Design review of the part built by this model. Coordinates are the model's own, in mm. A direction names the side the tool comes from. Give positions to 0.01 mm unless a question says otherwise; leave off trailing zeros. Write each loop counter-clockwise with the first axis right and the second up, starting at its lowest first coordinate (ties: lowest second). Pieces come first, ordered by that corner, then holes. Notation, with made-up numbers: (62.25, 79) -> (73.25, 79) arc R19 cw to (73.25, 114) -> close; hole circle Ø2 at (38.25, 38). An arc over 180 degrees is marked (long way). Use CSV: the item, a comma, the result in double quotes.
```python
from build123d import *

# Parameters (mm, degrees)
CHAMFER1_SIZE           = 0.5
CUT_EXTRUDE1_REACH      = 21.596
CUT_EXTRUDE1_END_RADIUS = 8
SKETCH2_R               = 1.5
CUT_EXTRUDE2_REACH      = 21.596
CUT_EXTRUDE2_END_RADIUS = 8
SKETCH3_R               = 1.5


with BuildPart() as part:
    # Sketch1 → Revolve1 (revolve)
    with BuildSketch(Plane.XY, mode=Mode.PRIVATE) as revolve1_sk:
        Polygon((-4, 0), (-4, 16), (-8, 16), (-8, 15), (-6.1, 15), (-6.1, 7), (-8, 7), (-8, 0), align=None)
    revolve(revolve1_sk.sketch.rotate(Axis((0, 0, 0), (0, 1, 0)), 270), axis=Axis((0, 0, 0), (0, 1, 0)))

    # Chamfer1
    chamfer1_edges = [part.edges().sort_by_distance(p)[0] for p in [
        (0, 0, 8),
    ]]
    chamfer(chamfer1_edges, length=CHAMFER1_SIZE)

    # Cut-Extrude1: up to this cylinder (the profile starts inside it)
    cut_extrude1_end = Plane(origin=(0, 3.5, 0), z_dir=(0, -1, 0)) * Cylinder(CUT_EXTRUDE1_END_RADIUS, 60.192, mode=Mode.PRIVATE)
    # Sketch2 → Cut-Extrude1 (cut, up to the surface)
    with BuildSketch(Plane.XY, mode=Mode.PRIVATE) as cut_extrude1_sk1:
        with Locations((0, 3.5)):
            Circle(SKETCH2_R)
    cut_extrude1_tool1 = extrude(cut_extrude1_sk1.sketch, amount=-CUT_EXTRUDE1_REACH, mode=Mode.PRIVATE) & cut_extrude1_end
    add(cut_extrude1_tool1.solids().sort_by_distance((0, 3.5, 0))[0], mode=Mode.SUBTRACT)

    # Cut-Extrude2: up to this cylinder (the profile starts inside it)
    cut_extrude2_end = Plane(origin=(0, 3.5, 0), z_dir=(0, -1, 0)) * Cylinder(CUT_EXTRUDE2_END_RADIUS, 60.192, mode=Mode.PRIVATE)
    # Sketch3 → Cut-Extrude2 (cut, up to the surface)
    with BuildSketch(Plane(origin=(0, 0, 0), x_dir=(0, 0, -1), z_dir=(1, 0, 0)), mode=Mode.PRIVATE) as cut_extrude2_sk1:
        with Locations((0, 3.5)):
            Circle(SKETCH3_R)
    cut_extrude2_tool1 = extrude(cut_extrude2_sk1.sketch, amount=-CUT_EXTRUDE2_REACH, mode=Mode.PRIVATE) & cut_extrude2_end
    add(cut_extrude2_tool1.solids().sort_by_distance((0, 3.5, 0))[0], mode=Mode.SUBTRACT)


solid = part.part
```
(1) Take a section at C-C (y = 3.5). Write out the cut boundary in (x, z).
Established:
outline,"(-7.86, -1.5) arc R8 ccw to (-1.5, -7.86) -> (-1.5, -3.71) arc R4 cw to (-3.71, -1.5) -> close; (-7.86, 1.5) -> (-3.71, 1.5) arc R4 cw (long way) to (1.5, -3.71) -> (1.5, -7.86) arc R8 ccw (long way) to start"
(2) For line 1 along X through (y, z) = (6, 0); line 2 along Y through (x, z) = (-4.25, 4.75); line 3 along Y through (x, z) = (-5, 0), list the stretches that pass through material, from the lowest coordinate up. Write a range as [from, to].
Established:
line 1,"x = [-8, -4], [4, 8]"
line 2,"y = [0, 7], [15, 16]"
line 3,"y = [0, 2], [5, 16]"
(3) Mouldability with a two-part tool opening along X and no side actions: class faces 4 (the face through (6, 15, 2)), 5 (the face through (3.71, 10.94, 4.84)), 6 (the face through (3.905, 8.112, 0.867)), 7 (the face through (-1.5, 3.57, -5.82)) as +X half, -X half, draft (parallel to the pull), parting line (faces both ways), or undercut.
Established:
face 4,"draft"
face 5,"parting line"
face 6,"undercut"
face 7,"undercut"
(4) Tool access review of faces 1 (the face through (7.81, 3.7, 1.73)), 2 (the face through (6, 7, -2)), 3 (the face through (-5.83, 3.57, 1.5)): name each direction out of +Z, -Z, +X, -X, +Y, -Y from which nothing blocks a thin tool from reaching the whole face with its end or side.
Established:
face 1,"+Y, -Y"
face 2,"none"
face 3,"-X"
(5) Take a section at A-A (z = 0). Write out the cut boundary in (x, y).
Established:
outline,"(-8, 0.5) -> (-7.5, 0) -> (-4, 0) -> (-4, 2) -> (-8, 2) -> close; (-8, 5) -> (-4, 5) -> (-4, 16) -> (-8, 16) -> (-8, 15) -> (-6.1, 15) -> (-6.1, 7) -> (-8, 7) -> close; (4, 0) -> (7.5, 0) -> (8, 0.5) -> (8, 7) -> (6.1, 7) -> (6.1, 15) -> (8, 15) -> (8, 16) -> (4, 16) -> close"
(6) Take a section at D-D (y = 8.5). Write out the cut boundary in (x, z), then the cut area to 3 significant figures.
Established:
outline,"circle Ø12.2 at (0, 0); hole circle Ø8 at (0, 0)"
area,"66.6 mm2"
(7) Take a section at B-B (x = 0). Write out the cut boundary in (y, z).
Established:
outline,"(0, -7.5) -> (0.5, -8) -> (2, -8) -> (2, -4) -> (0, -4) -> close; (0, 4) -> (16, 4) -> (16, 8) -> (15, 8) -> (15, 6.1) -> (7, 6.1) -> (7, 8) -> (0.5, 8) -> (0, 7.5) -> close; (5, -8) -> (7, -8) -> (7, -6.1) -> (15, -6.1) -> (15, -8) -> (16, -8) -> (16, -4) -> (5, -4) -> close"
(8) Clearance check with flat-ended pins moving along their axes: pin 1 (4 mm diameter, centred on y = 5, z = -5.5, fed in from -X); pin 2 (1.5 mm diameter, centred on x = -4.5, y = 6.5, fed in from -Z); pin 3 (2.5 mm diameter, centred on x = 0, y = 3.5, fed in from -Z); pin 4 (6.5 mm diameter, centred on x = 0, z = 0, fed in from -Y). State where each tip first meets the part, or that it passes through.
Established:
pin 1,"stops at x = -7.19"
pin 2,"stops at z = -7.07"
pin 3,"stops at z = 3.8"
pin 4,"passes through"
